from build123d import *

# Parameters (mm, degrees)
SKETCH1_W           = 38.1
SKETCH1_H           = 25.4
SKETCH1_W_2         = 31.75
SKETCH1_H_2         = 19.05
BOSS_EXTRUDE1_DEPTH = 184.15
CUT_EXTRUDE1_REACH  = 188.867
CUT_EXTRUDE2_REACH  = 188.867
SKETCH3_R           = 4.7625
SKETCH3_R_2         = 2.54


with BuildPart() as part:
    # Sketch1 → Boss-Extrude1 (new body)
    with BuildSketch(Plane.XY):
        Rectangle(SKETCH1_W, SKETCH1_H)
        Rectangle(SKETCH1_W_2, SKETCH1_H_2, mode=Mode.SUBTRACT)
    extrude(amount=BOSS_EXTRUDE1_DEPTH)

    # Cut-Extrude1: up to this face of the body (flat: up to its plane)
    cut_extrude1_end = Plane(part.part.faces().sort_by_distance((0, -12.7, 92.075))[0])
    # Sketch2 → Cut-Extrude1 (cut, up to the picked face)
    with BuildSketch(Plane(origin=(0, 12.7, 0), x_dir=(1, 0, 0), z_dir=(0, 1, 0)), mode=Mode.PRIVATE) as cut_extrude1_sk1:
        Polygon((19.05, -184.15), (-19.05, -167.977509502), (-19.05, -184.15), align=None)
    cut_extrude1_tool1 = split(extrude(cut_extrude1_sk1.sketch, amount=-CUT_EXTRUDE1_REACH, mode=Mode.PRIVATE), bisect_by=cut_extrude1_end, keep=Keep.BOTH, mode=Mode.PRIVATE)
    add(cut_extrude1_tool1.solids().sort_by(Axis((-6.35, 12.7, 178.75917), (0, -1, 0)))[0], mode=Mode.SUBTRACT)

    # Cut-Extrude2: up to this face of the body (flat: up to its plane)
    cut_extrude2_end = Plane(part.part.faces().sort_by_distance((0.291642408, -12.7, 88.093774804))[0])
    # Sketch3 → Cut-Extrude2 (cut, up to the picked face)
    with BuildSketch(Plane(origin=(0, 12.7, 0), x_dir=(1, 0, 0), z_dir=(0, 1, 0)), mode=Mode.PRIVATE) as cut_extrude2_sk1:
        with Locations(Location((-4.7625, -31.75, 0), (0, 0, 270))):
            Circle(SKETCH3_R)
    cut_extrude2_tool1 = split(extrude(cut_extrude2_sk1.sketch, amount=-CUT_EXTRUDE2_REACH, mode=Mode.PRIVATE), bisect_by=cut_extrude2_end, keep=Keep.BOTH, mode=Mode.PRIVATE)
    # Sketch3 → Cut-Extrude2 (cut, up to the picked face)
    with BuildSketch(Plane(origin=(0, 12.7, 0), x_dir=(1, 0, 0), z_dir=(0, 1, 0)), mode=Mode.PRIVATE) as cut_extrude2_sk2:
        with Locations(Location((-12.906854663, -54.126430532, 0), (0, 0, 270))):
            Circle(SKETCH3_R_2)
    cut_extrude2_tool2 = split(extrude(cut_extrude2_sk2.sketch, amount=-CUT_EXTRUDE2_REACH, mode=Mode.PRIVATE), bisect_by=cut_extrude2_end, keep=Keep.BOTH, mode=Mode.PRIVATE)
    # Sketch3 → Cut-Extrude2 (cut, up to the picked face)
    with BuildSketch(Plane(origin=(0, 12.7, 0), x_dir=(1, 0, 0), z_dir=(0, 1, 0)), mode=Mode.PRIVATE) as cut_extrude2_sk3:
        with Locations(Location((3.381854663, -9.373569468, 0), (0, 0, 270))):
            Circle(SKETCH3_R_2)
    cut_extrude2_tool3 = split(extrude(cut_extrude2_sk3.sketch, amount=-CUT_EXTRUDE2_REACH, mode=Mode.PRIVATE), bisect_by=cut_extrude2_end, keep=Keep.BOTH, mode=Mode.PRIVATE)
    # Sketch3 → Cut-Extrude2 (cut, up to the picked face)
    with BuildSketch(Plane(origin=(0, 12.7, 0), x_dir=(1, 0, 0), z_dir=(0, 1, 0)), mode=Mode.PRIVATE) as cut_extrude2_sk4:
        with Locations(Location((10.543879956, -49.991433302, 0), (0, 0, 270))):
            Circle(SKETCH3_R_2)
    cut_extrude2_tool4 = split(extrude(cut_extrude2_sk4.sketch, amount=-CUT_EXTRUDE2_REACH, mode=Mode.PRIVATE), bisect_by=cut_extrude2_end, keep=Keep.BOTH, mode=Mode.PRIVATE)
    add(cut_extrude2_tool1.solids().sort_by(Axis((-4.7625, 12.7, 31.75), (0, -1, 0)))[0], mode=Mode.SUBTRACT)
    add(cut_extrude2_tool2.solids().sort_by(Axis((-12.906855, 12.7, 54.126431), (0, -1, 0)))[0], mode=Mode.SUBTRACT)
    add(cut_extrude2_tool3.solids().sort_by(Axis((3.381855, 12.7, 9.373569), (0, -1, 0)))[0], mode=Mode.SUBTRACT)
    add(cut_extrude2_tool4.solids().sort_by(Axis((10.54388, 12.7, 49.991433), (0, -1, 0)))[0], mode=Mode.SUBTRACT)


solid = part.part
Check sheet for the modelled part. Datum: model origin and axes. Units: mm. A direction names the side the tool comes from. Coordinates: 2 decimals unless noted, no trailing zeros. Loops run counter-clockwise (first coordinate to the right, second up) from the corner with the lowest first, then second, coordinate; pieces in that order, holes last. Notation, with made-up numbers: (39, 8) -> (48, 8) arc R20 cw to (48, 12) -> close; hole circle Ø8 at (18, 54.25). An arc over 180 degrees is marked (long way). Answer in a Markdown table with one row per item.
1. Material ranges on line 1 along X through (y, z) = (-0.25, 74) (3 decimals); line 2 along Y through (x, z) = (-14, 17.5) (3 decimals); line 3 along X through (y, z) = (10.8, 31.75) (3 decimals), recorded low to high. Write a range as [from, to].
Check values:
| item | result |
|---|---|
| line 1 | x = [-19.05, -15.875], [15.875, 19.05] |
| line 2 | y = [-12.7, -9.525], [9.525, 12.7] |
| line 3 | x = [-19.05, -9.525], [0, 19.05] |
2. Access from +Z, -Z, +X, -X, +Y, -Y to the whole of each face (thin tool, end or side, straight path). Record for faces 5 (the face through (19.05, 0, 91)), 6 (the face through (0, -9.525, 90)).
Check values:
| item | result |
|---|---|
| face 5 | +Z, -Z, +X, +Y, -Y |
| face 6 | +Z, -Z |
3. Sectioned sample at D-D, the plane z = 121.5. Record the boundary of the cut face in (x, y) (3 decimals), then the cut area to 3 significant figures.
Check values:
| item | result |
|---|---|
| outline | (-19.05, -12.7) -> (19.05, -12.7) -> (19.05, 12.7) -> (-19.05, 12.7) -> close; hole (-15.875, -9.525) -> (15.875, -9.525) -> (15.875, 9.525) -> (-15.875, 9.525) -> close |
| area | 363 mm2 |
4. Sectioned sample at C-C, the plane x = -2. Record the boundary of the cut face in (y, z) (3 decimals), then the cut area to 3 significant figures.
Check values:
| item | result |
|---|---|
| outline | (-12.7, 0) -> (-9.525, 0) -> (-9.525, 27.871) -> (-12.7, 27.871) -> close; (-12.7, 35.629) -> (-9.525, 35.629) -> (-9.525, 175.215) -> (-12.7, 175.215) -> close; (9.525, 0) -> (12.7, 0) -> (12.7, 27.871) -> (9.525, 27.871) -> close; (9.525, 35.629) -> (12.7, 35.629) -> (12.7, 175.215) -> (9.525, 175.215) -> close |
| area | 1,060 mm2 |
5. Release check for a two-part mould opening along Y. For faces 1 (the face through (0, 12.7, 91)), 2 (the face through (0, -12.7, 91)), 3 (the face through (11.307, 11.135, 52.414)), 4 (the face through (0, 9.525, 90)) record: released by +Y, released by -Y, zero draft, split by the parting line, or undercut.
Check values:
| item | result |
|---|---|
| face 1 | released by +Y |
| face 2 | released by -Y |
| face 3 | zero draft |
| face 4 | undercut |
6. Sectioned sample at A-A, the plane z = 31.75. Record the boundary of the cut face in (x, y) (3 decimals).
Check values:
| item | result |
|---|---|
| outline | (-19.05, -12.7) -> (-9.525, -12.7) -> (-9.525, -9.525) -> (-15.875, -9.525) -> (-15.875, 9.525) -> (-9.525, 9.525) -> (-9.525, 12.7) -> (-19.05, 12.7) -> close; (0, -12.7) -> (19.05, -12.7) -> (19.05, 12.7) -> (0, 12.7) -> (0, 9.525) -> (15.875, 9.525) -> (15.875, -9.525) -> (0, -9.525) -> close |
